Design review of the part built by this model. Coordinates are the model's own, in mm. A direction names the side the tool comes from. Give positions to 0.01 mm unless a question says otherwise; leave off trailing zeros. Write each loop counter-clockwise with the first axis right and the second up, starting at its lowest first coordinate (ties: lowest second). Pieces come first, ordered by that corner, then holes.
```python
from build123d import *

# Parameters (mm, degrees)
SKETCH_2_R             = 6.5
EXTRUDE_1_DEPTH        = 5
SKETCH_3_R             = 9
EXTRUDE_2_DEPTH        = 6.5
SKETCH_4_R             = 3
CUT_EXTRUDE_1_DEPTH    = 18
EXTRUDE_3_REACH        = 37.767
EXTRUDE_3_END_RADIUS   = 9
SKETCH_7_R             = 5
SKETCH_8_R             = 9
CUT_EXTRUDE_6_DEPTH    = 2
SKETCH_11_R            = 9
SKETCH_11_R_2          = 4.5
CUT_EXTRUDE_8_DEPTH    = 1.125
HOLE_WIZARD_M6_3_D     = 5
HOLE_WIZARD_M6_3_DEPTH = 17
HOLE_WIZARD_M6_3_TIP   = 1.502151548


with BuildPart() as part:
    # Sketch 2 → Extrude 1 (new body)
    with BuildSketch(Plane.XY):
        Circle(SKETCH_2_R)
    extrude(amount=EXTRUDE_1_DEPTH)



with BuildPart() as body_2:
    # Sketch 3 → Extrude 2 (new, symmetric)
    with BuildSketch(Plane(origin=(0, 0, 0), x_dir=(1, 0, 0), z_dir=(0, 1, 0))):
        with Locations(Location((0, -30, 0), (0, 0, 90))):
            Circle(SKETCH_3_R)
    extrude(amount=EXTRUDE_2_DEPTH, both=True)

    # Sketch 4 → Cut-Extrude 1 (cut)
    with BuildSketch(Plane(origin=(0, 6.5, 0), x_dir=(1, 0, 0), z_dir=(0, 1, 0))):
        with Locations(Location((0, -30, 0), (0, 0, 270))):
            Circle(SKETCH_4_R)
    extrude(amount=-CUT_EXTRUDE_1_DEPTH, mode=Mode.SUBTRACT)


with BuildPart() as part_1:
    add(part.part)

    add(body_2.part)  # Extrude 3 merges body 2
    # Extrude 3: up to this cylinder (the profile starts outside it)
    extrude_3_end = Plane(origin=(0, 0, 30), z_dir=(0, -1, 0)) * Cylinder(EXTRUDE_3_END_RADIUS, 94.534, mode=Mode.PRIVATE)
    # Sketch 7 → Extrude 3 (add, up to the surface)
    with BuildSketch(Plane.XY.offset(5), mode=Mode.PRIVATE) as extrude_3_sk1:
        with Locations(Location((0, 0, 0), (0, 0, 180))):
            Circle(SKETCH_7_R)
    extrude_3_tool1 = extrude(extrude_3_sk1.sketch, amount=EXTRUDE_3_REACH, mode=Mode.PRIVATE) - extrude_3_end
    add(extrude_3_tool1.solids().sort_by_distance((0, 0, 5))[0])

    # Sketch 8 → Cut-Extrude 6 (cut)
    with BuildSketch(Plane(origin=(0, 6.5, 0), x_dir=(1, 0, 0), z_dir=(0, 1, 0))):
        with Locations(Location((0, -30, 0), (0, 0, 75.985881611))):
            Circle(SKETCH_8_R)
    cut_extrude_6 = extrude(amount=-CUT_EXTRUDE_6_DEPTH, mode=Mode.SUBTRACT)

    # Mirror 2: Cut-Extrude 6 across plane
    add(cut_extrude_6.mirror(Plane.ZX), mode=Mode.SUBTRACT)

    # Sketch 11 → Cut-Extrude 8 (cut)
    with BuildSketch(Plane(origin=(0, 4.5, 0), x_dir=(1, 0, 0), z_dir=(0, 1, 0))):
        with Locations((0, -30)):
            Circle(SKETCH_11_R)
        with Locations(Location((0, -30, 0), (0, 0, 270))):
            Circle(SKETCH_11_R_2, mode=Mode.SUBTRACT)
    cut_extrude_8 = extrude(amount=-CUT_EXTRUDE_8_DEPTH, mode=Mode.SUBTRACT)

    # Mirror 3: Cut-Extrude 8 across plane
    add(cut_extrude_8.mirror(Plane.ZX), mode=Mode.SUBTRACT)

    # Hole Wizard M6 _3
    with Locations(Plane(origin=(0, 0, 0), x_dir=(-1, 0, 0), z_dir=(0, 0, -1))):
        with Locations((0, 0)):
            Hole(HOLE_WIZARD_M6_3_D / 2, depth=HOLE_WIZARD_M6_3_DEPTH)
            with Locations((0, 0, -(HOLE_WIZARD_M6_3_DEPTH + HOLE_WIZARD_M6_3_TIP / 2))):  # 118° drill point
                Cone(0, HOLE_WIZARD_M6_3_D / 2, HOLE_WIZARD_M6_3_TIP, mode=Mode.SUBTRACT)


solid = part_1.part
```
(1) Clearance check with flat-ended pins moving along their axes: P1, Ø4.5, axis at x = -1, z = 29.5, coming from the -Y side; P2, Ø8, axis at x = 4, z = 11.5, coming from the -Y side; P3, Ø3, axis at x = -6, z = 34, coming from the -Y side (3 decimals). State where each tip first meets the part, or that it passes through.
Resolved:
P1: stops at y = -4.5
P2: stops at y = -5
P3: stops at y = -3.375
(2) Mouldability with a two-part tool opening along X and no side actions: class faces 1 (the face through (-0.54, -2.44, 8.62)), 2 (the face through (2, -5, 5)), 3 (the face through (0, 4, 21)), 4 (the face through (1.352, 3.945, 34.292)) as pulls with the +X half, pulls with the -X half, needs draft (parallel to the pull), parting line crosses it, or undercut.
Resolved:
face 1: undercut
face 2: needs draft
face 3: undercut
face 4: parting line crosses it
(3) Consider section C-C, the plane y = 5.5. Give the boundary of the cut face in (x, z), then the cut area to 3 significant figures.
Resolved:
outline: (-3.46, 0) - (3.46, 0) - (3.46, 5) - (-3.46, 5) - close
area: 34.6 mm2
(4) To check wall thickness, follow L1, parallel to Z at x = -0.75, y = 3.75; L2, parallel to Y at x = 2.5, z = 26 (3 decimals); L3, parallel to X at y = -0.25, z = 30. State the ranges of each line that lie inside material, in increasing order.
Resolved:
L1: z = 0 to 21.03, 25.56 to 27.1, 32.9 to 34.44
L2: y = -3.375 to 3.375
L3: x = -9 to -3, 3 to 9
(5) Consider section B-B, the plane z = 17.5. Give the boundary of the cut face in (x, y), then the cut area to 3 significant figures.
Resolved:
outline: circle Ø10 at (0, 0); hole circle Ø3.34 at (0, 0)
area: 69.8 mm2
(6) Consider section D-D, the plane x = 7. Give the boundary of the cut face in (y, z) (3 decimals).
Resolved:
outline: (-3.375, 24.343) - (3.375, 24.343) - (3.375, 35.657) - (-3.375, 35.657) - close
(7) Consider section A-A, the plane z = 30. Give the boundary of the cut face in (x, y) (3 decimals).
Resolved:
outline: (-9, -3.375) - (-4.5, -3.375) - (-4.5, -4.5) - (-3, -4.5) - (-3, 4.5) - (-4.5, 4.5) - (-4.5, 3.375) - (-9, 3.375) - close; (3, -4.5) - (4.5, -4.5) - (4.5, -3.375) - (9, -3.375) - (9, 3.375) - (4.5, 3.375) - (4.5, 4.5) - (3, 4.5) - close
(8) Tool access review of faces 5 (the face through (5, 0, 14)), 6 (the face through (1.352, -3.945, 34.292)), 7 (the face through (2, -4.5, 27)), 8 (the face through (2, 4.5, 27)): name each direction out of +Z, -Z, +X, -X, +Y, -Y from which nothing blocks a thin tool from reaching the whole face with its end or side.
Resolved:
face 5: none
face 6: -Y
face 7: +Z, +X, -X, -Y
face 8: +Z, +X, -X, +Y
